```python
from build123d import *

# Parameters (mm, degrees)
RECTANGULAR_TUBE_3_X_2_X_0_25_1_DEPTH = 152.4
F_1_2_CLEARANCE_HOLE1_D               = 13.49248


with BuildPart() as part:
    # Sketch16 → Rectangular tube 3 X 2 X 0.25(1) (new body)
    with BuildSketch(Plane.ZY.offset(-76.2)):
        with BuildLine():
            Line((-33.3375, -12.7), (33.3375, -12.7))
            ThreePointArc((33.3375, -12.7), (36.705096045, -11.305096045), (38.1, -7.9375))
            Line((38.1, -7.9375), (38.1, 7.9375))
            ThreePointArc((38.1, 7.9375), (36.705096045, 11.305096045), (33.3375, 12.7))
            Line((33.3375, 12.7), (-33.3375, 12.7))
            ThreePointArc((-33.3375, 12.7), (-36.705096045, 11.305096045), (-38.1, 7.9375))
            Line((-38.1, 7.9375), (-38.1, -7.9375))
            ThreePointArc((-38.1, -7.9375), (-36.705096045, -11.305096045), (-33.3375, -12.7))
        make_face()
        with BuildLine():
            Line((-33.3375, -9.652), (33.3375, -9.652))
            ThreePointArc((33.3375, -9.652), (34.549834576, -9.149834576), (35.052, -7.9375))
            Line((35.052, -7.9375), (35.052, 7.9375))
            ThreePointArc((35.052, 7.9375), (34.549834576, 9.149834576), (33.3375, 9.652))
            Line((33.3375, 9.652), (-33.3375, 9.652))
            ThreePointArc((-33.3375, 9.652), (-34.549834576, 9.149834576), (-35.052, 7.9375))
            Line((-35.052, 7.9375), (-35.052, -7.9375))
            ThreePointArc((-35.052, -7.9375), (-34.549834576, -9.149834576), (-33.3375, -9.652))
        make_face(mode=Mode.SUBTRACT)
    extrude(amount=RECTANGULAR_TUBE_3_X_2_X_0_25_1_DEPTH)

    # 1/2 Clearance Hole1 (through all)
    with Locations(Plane(origin=(0, 12.7, 0), x_dir=(1, 0, 0), z_dir=(0, 1, 0))):
        with Locations((-50.8, 0), (50.8, 0)):
            Hole(F_1_2_CLEARANCE_HOLE1_D / 2)


solid = part.part
```
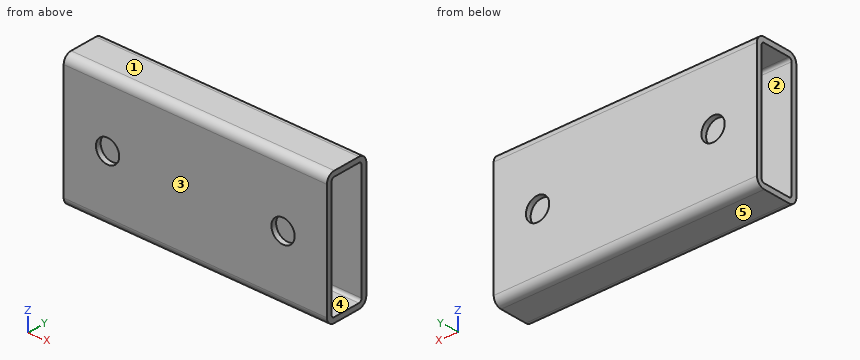
The model under review builds one solid part; all positions refer to its coordinate system, in mm. Face numbers are marked on the shaded views. A direction names the side the tool comes from. Give positions to 0.01 mm unless a question says otherwise; leave off trailing zeros. Loops run counter-clockwise (first coordinate to the right, second up) from the corner with the lowest first, then second, coordinate; pieces in that order, holes last. Notation, with made-up numbers: (53, 20.5) - (105, 20.5) arc R17 ccw to (105, 43.5) - close; hole circle Ø1 at (53, 75). An arc over 180 degrees is marked (long way). Answer as a JSON object with one key per item and string values.
Q1. Add section A-A on y = 3.5. State the section outline as (x, z) points, plus the area to 3 significant figures.
Worked out:
{"outline": "(-76.2, -38.1) - (76.2, -38.1) - (76.2, -35.05) - (-76.2, -35.05) - close; (-76.2, 35.05) - (76.2, 35.05) - (76.2, 38.1) - (-76.2, 38.1) - close", "area": "929 mm^2"}
Q2. Add section B-B on x = -14.5. State the section outline as (y, z) points (1 decimal).
Worked out:
{"outline": "(-12.7, -33.3) arc R4.8 ccw to (-7.9, -38.1) - (7.9, -38.1) arc R4.8 ccw to (12.7, -33.3) - (12.7, 33.3) arc R4.8 ccw to (7.9, 38.1) - (-7.9, 38.1) arc R4.8 ccw to (-12.7, 33.3) - close; hole (-9.7, -33.3) arc R1.7 ccw to (-7.9, -35.1) - (7.9, -35.1) arc R1.7 ccw to (9.7, -33.3) - (9.7, 33.3) arc R1.7 ccw to (7.9, 35.1) - (-7.9, 35.1) arc R1.7 ccw to (-9.7, 33.3) - close"}
Q3. Add section D-D on x = -50.8. State the section outline as (y, z) points (1 decimal), plus the area to 3 significant figures.
Worked out:
{"outline": "(-12.7, -33.3) arc R4.8 ccw to (-7.9, -38.1) - (7.9, -38.1) arc R4.8 ccw to (12.7, -33.3) - (12.7, -6.7) - (9.7, -6.7) - (9.7, -33.3) arc R1.7 cw to (7.9, -35.1) - (-7.9, -35.1) arc R1.7 cw to (-9.7, -33.3) - (-9.7, -6.7) - (-12.7, -6.7) - close; (-12.7, 6.7) - (-9.7, 6.7) - (-9.7, 33.3) arc R1.7 cw to (-7.9, 35.1) - (7.9, 35.1) arc R1.7 cw to (9.7, 33.3) - (9.7, 6.7) - (12.7, 6.7) - (12.7, 33.3) arc R4.8 ccw to (7.9, 38.1) - (-7.9, 38.1) arc R4.8 ccw to (-12.7, 33.3) - close", "area": "483 mm^2"}
Q4. To check wall thickness, follow line 1 along Y through (x, z) = (-55, 25.5); line 2 along Z through (x, y) = (22.5, 4.5); line 3 along Z through (x, y) = (-50.8, 11.7). State the ranges of each line that lie inside material, in increasing order.
Worked out:
{"line 1": "y = -12.7 to -9.65, 9.65 to 12.7", "line 2": "z = -38.1 to -35.05, 35.05 to 38.1", "line 3": "z = -36.26 to -6.75, 6.75 to 36.26"}
Q5. Mouldability with a two-part tool opening along Y and no side actions: class the marked faces 1, 2 and 3 as +Y half, -Y half, draft (parallel to the pull), parting line (faces both ways), or undercut.
Worked out:
{"face 1": "draft", "face 2": "undercut", "face 3": "-Y half"}
Q6. Add section C-C on z = 0. State the section outline as (x, y) points, plus the area to 3 significant figures.
Worked out:
{"outline": "(-76.2, -12.7) - (-57.55, -12.7) - (-57.55, -9.65) - (-76.2, -9.65) - close; (-76.2, 9.65) - (-57.55, 9.65) - (-57.55, 12.7) - (-76.2, 12.7) - close; (-44.05, -12.7) - (44.05, -12.7) - (44.05, -9.65) - (-44.05, -9.65) - close; (-44.05, 9.65) - (44.05, 9.65) - (44.05, 12.7) - (-44.05, 12.7) - close; (57.55, -12.7) - (76.2, -12.7) - (76.2, -9.65) - (57.55, -9.65) - close; (57.55, 9.65) - (76.2, 9.65) - (76.2, 12.7) - (57.55, 12.7) - close", "area": "765 mm^2"}
Q7. For the marked faces 4 and 5, list the 3-axis set-ups (+Z, -Z, +X, -X, +Y, -Y) from which the entire face can be reached by the end or side of a thin tool; tool diameter is ignored.
Worked out:
{"face 4": "+X, -X", "face 5": "-Z, +X, -X, +Y, -Y"}
